from build123d import *

# Parameters (mm, degrees)
F0_W          = 90
F0_H          = 35
F1_DEPTH      = 3
F2_W          = 90
F2_H          = 23
F3_DEPTH      = 2
F5_DEPTH      = 45
F5_DEPTH_BACK = 45
F7_START      = 3
F6_W          = 86
F6_H          = 33
F7_DEPTH      = 32.9
F8_R          = 12.5
F8_R_2        = 8
F9_DEPTH      = 3


with BuildPart() as f1:
    # F0 (on Top) → F1 (new body)
    with BuildSketch(Plane.XY):
        with Locations((0, -17.5)):
            Rectangle(F0_W, F0_H)
    extrude(amount=F1_DEPTH)

    # F2 (on Front) → F3 (join)
    with BuildSketch(Plane.XZ):
        with Locations((0, 11.5)):
            Rectangle(F2_W, F2_H)
    extrude(amount=F3_DEPTH)

    # F4 (on Right) → F5 (join, two sides)
    with BuildSketch(Plane.YZ) as f5_sk:
        with BuildLine():
            Line((-18.3083641247, 0), (0, 0))
            Line((0, 0), (0, 18.3083641247))
            ThreePointArc((0, 18.3083641247), (-12.945968425, 12.945968425), (-18.3083641247, 0))
        make_face()
    extrude(amount=F5_DEPTH)
    extrude(f5_sk.sketch, amount=-F5_DEPTH_BACK)

    # F6 (on Top) → F7 (cut)
    with BuildSketch(Plane.XY.offset(F7_START)):
        with Locations((0, -18.5)):
            Rectangle(F6_W, F6_H)
    extrude(amount=F7_DEPTH, mode=Mode.SUBTRACT)

    # F8 (on Top) → F9 (cut)
    with BuildSketch(Plane.XY):
        with Locations((18.9312342554, -17.8462527692)):
            Circle(F8_R)
        with Locations((-21.9019707292, -17.8462527692)):
            Circle(F8_R_2)
    extrude(amount=F9_DEPTH, mode=Mode.SUBTRACT)


solid = f1.part
Source: CAD feature listing. Evaluate the final solid. Frame: model axes, mm. A direction names the side the tool comes from. Coordinates: 2 decimals unless noted, no trailing zeros. Order: outer loops, then holes, each group sorted by start corner. A loop starts at its lowest first (then second) coordinate and runs counter-clockwise, first axis right, second up. Notation, with made-up numbers: M 53.5,-37 L 99.5,-37 A33 ccw 99.5,-5 Z; hole C 62,71 d5. An arc over 180 degrees is marked long. Write each question's results on one line, items separated by ' | '. Start each with the question number.
1. Section A-A, the plane y = -23. Return the cut outline in (x, z).
2. Draft query along X for faces 1 (the face through (-27.8, -12.44, 1.48)), 2 (the face through (45, -10, 6)), 3 (the face through (-44.014, -12.463, 13.412)). Return one class per face: +X half, -X half, draft (parallel to the pull), parting line (faces both ways), or undercut.
3. Section D-D, the plane y = -29.5. Return the cut outline in (x, z), then the cut area to 3 significant figures.
4. Section B-B, the plane x = 21. Return the cut outline in (y, z).
5. Pin query (flat end, axial travel): pin 1 (6 mm diameter, centred on x = -18, z = 12.5, fed in from -Y); pin 2 (6 mm diameter, centred on x = -27.5, y = -17.5, fed in from +Z); pin 3 (14.5 mm diameter, centred on x = -21.9, y = -17.85, fed in from -Z). Return the tip coordinate at first contact, or that it passes through.
6. Material intervals for L1, parallel to X at y = -6, z = 7.5; L2, parallel to Z at x = -18, y = -28; L3, parallel to Y at x = 10.5, z = 15, sorted ascending.
7. Reachability of faces 4 (the face through (-1, -18, 3)), 5 (the face through (43.986, -12.463, 13.412)) from +Z, -Z, +X, -X, +Y, -Y: full face, straight path, thin tool, end or side. Return the list, or none.
8. Section C-C, the plane z = 16. Return the cut outline in (x, y).
Solution:
1) outline: M -45,0 L -28.02,0 L -28.02,3 L -45,3 Z; M -15.78,0 L 7.54,0 L 7.54,3 L -15.78,3 Z; M 30.32,0 L 45,0 L 45,3 L 30.32,3 Z
2) face 1: undercut | face 2: +X half | face 3: draft
3) outline: M -45,0 L 14.41,0 L 14.41,3 L -45,3 Z; M 23.45,0 L 45,0 L 45,3 L 23.45,3 Z | area: 243 mm²
4) outline: M -35,0 L -30.17,0 L -30.17,3 L -35,3 Z; M -5.52,0 L 0,0 L 0,23 L -2,23 L -2,3 L -5.52,3 Z
5) pin 1: y = -2 | pin 2: z = 3 | pin 3: through
6) L1: -45 to -43, 43 to 45 | L2: 0 to 3 | L3: -2 to 0
7) face 4: +Z, -Y | face 5: +Z, +X, -X, -Y
8) outline: M -45,-8.9 L -43,-8.9 L -43,-2 L 43,-2 L 43,-8.9 L 45,-8.9 L 45,0 L -45,0 Z
